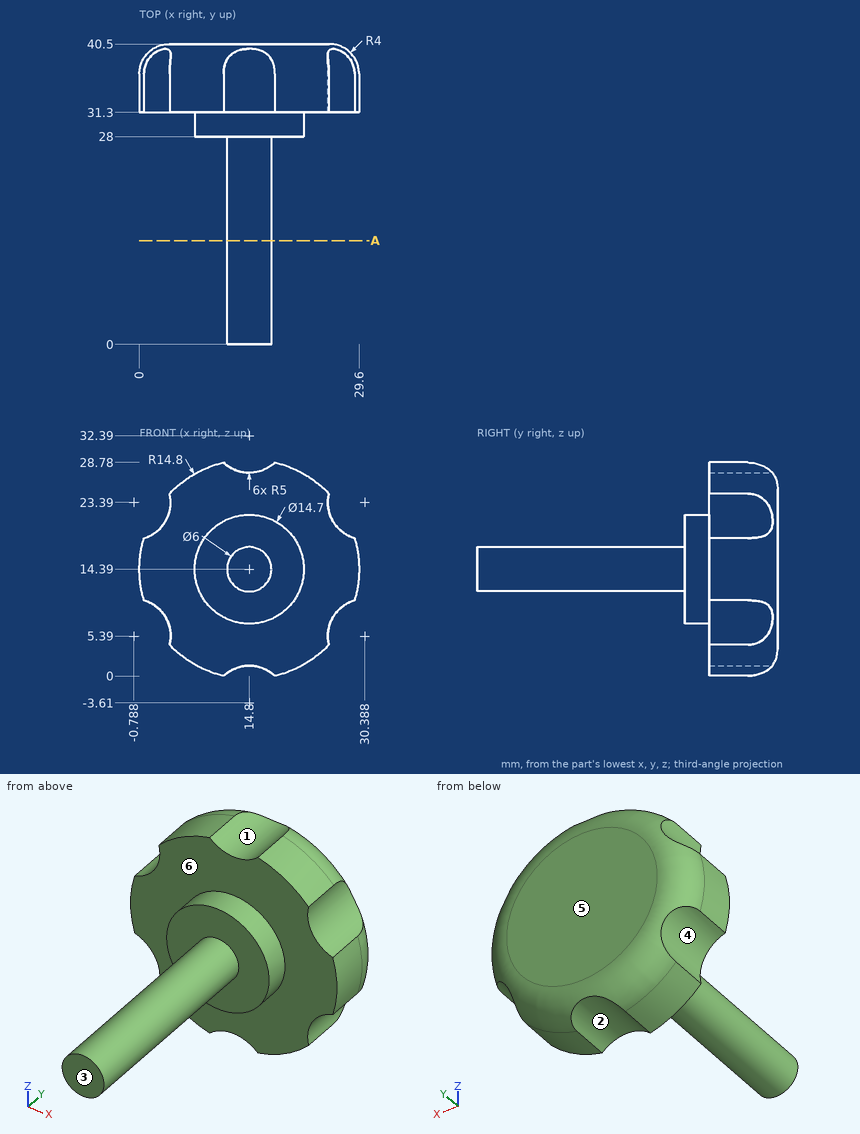
Check sheet for the drawn part. Datum: minimum x, y, z corner. Units: mm. A direction names the side the tool comes from. Give positions to 0.01 mm unless a question says otherwise; leave off trailing zeros. Write each loop counter-clockwise with the first axis right and the second up, starting at its lowest first coordinate (ties: lowest second). Pieces come first, ordered by that corner, then holes.
(1) Mould release check, pull along X, two halves, no side actions. Record for the marked faces 1, 2, 3 and 4: +X half, -X half, draft (parallel to the pull), parting line (faces both ways), or undercut.
(2) Gauge pin test, flat ends, axial feed: pin 1 (4 mm diameter, centred on y = 29, z = 23, fed in from -X) (1 decimal); pin 2 (3 mm diameter, centred on x = 17.5, y = 14.5, fed in from -Z); pin 3 (8 mm diameter, centred on x = 19, y = 8.5, fed in from +Z). Record the tip position at first contact, or that the pin passes through.
(3) Cross-section at A-A (y = 14). Enter the section's corners in (x, z), plus the area to 3 significant figures.
(4) Access from +Z, -Z, +X, -X, +Y, -Y to the whole of each face (thin tool, end or side, straight path). Record for the marked faces 5 and 6.
(5) Material ranges on line 1 (Y direction, x = 8.25, z = 11.5); line 2 (X direction, y = 36, z = 14.5); line 3 (Y direction, x = 20.5, z = 5.25), recorded low to high.
Worked out:
1. face 1: undercut
1. face 2: undercut
1. face 3: draft
1. face 4: -X half
2. pin 1: stops at x = 11.6
2. pin 2: stops at z = 11.64
2. pin 3: stops at z = 17.38
3. outline: circle Ø6 at (14.8, 14.39)
3. area: 28.3 mm2
4. face 5: +Z, -Z, +X, -X, +Y
4. face 6: -Y
5. line 1: y = 28 to 40.5
5. line 2: x = 0 to 29.6
5. line 3: y = 31.3 to 40.5
